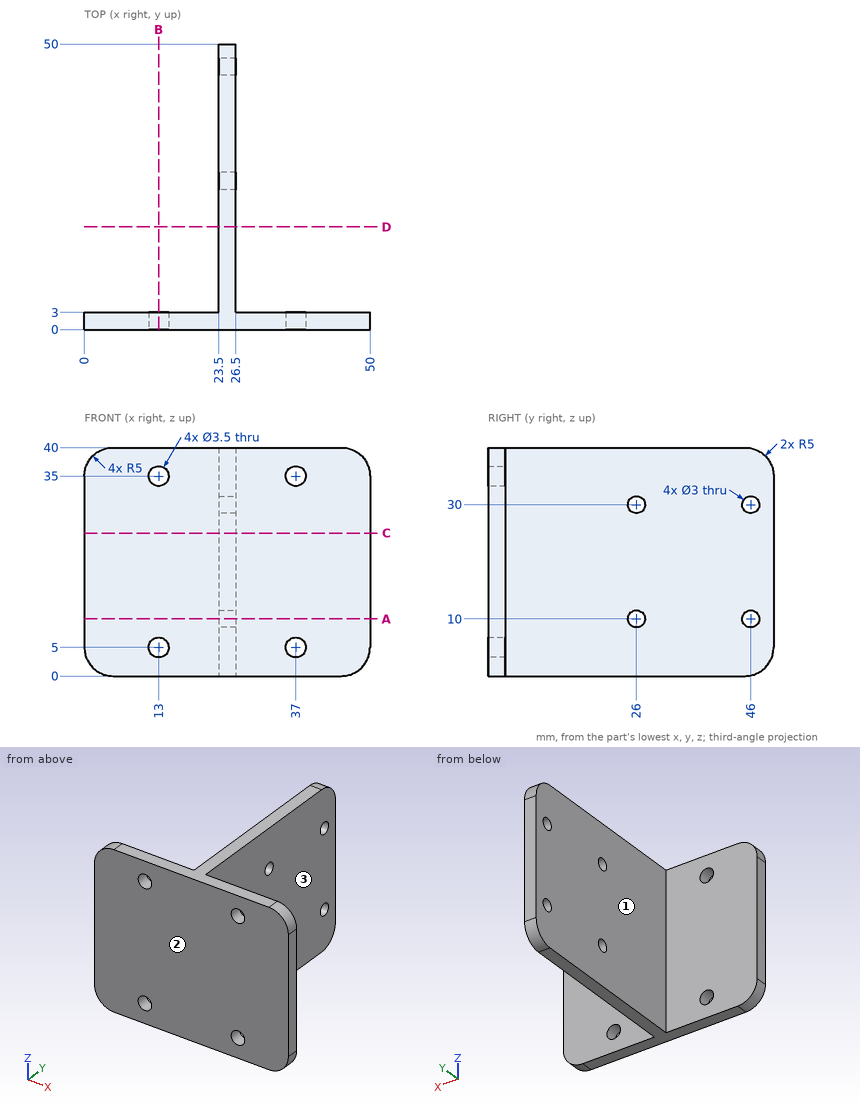
Job drawing, mm, ordinate dimensions from the low corner. One solid piece. A direction names the side the tool comes from. Give positions to 0.01 mm unless a question says otherwise; leave off trailing zeros. Loops run counter-clockwise (first coordinate to the right, second up) from the corner with the lowest first, then second, coordinate; pieces in that order, holes last.
Item 1: Slice it at B-B, the plane x = 13. List the corners of the cut face in (y, z), and give its area (3 significant figures).
Answers follow:
outline: (0, 0) - (3, 0) - (3, 3.25) - (0, 3.25) - close; (0, 6.75) - (3, 6.75) - (3, 33.25) - (0, 33.25) - close; (0, 36.75) - (3, 36.75) - (3, 40) - (0, 40) - close
area: 99.0 mm2
Item 2: Drill centre lines: line 1 (Y direction, x = 25, z = 30); line 2 (Y direction, x = 5, z = 13); line 3 (X direction, y = 40.5, z = 8.5). Where is each one in solid material? Low to high.
Answers follow:
line 1: y = 0 to 24.5, 27.5 to 44.5, 47.5 to 50
line 2: y = 0 to 3
line 3: x = 23.5 to 26.5
Item 3: Which spindle directions (+Z, -Z, +X, -X, +Y, -Y) get a long thin tool onto all of the face, cutting with end or side? Do the marked faces 1, 2 and 3. Say none if no direction does.
Answers follow:
face 1: +Z, -Z, -X, +Y
face 2: +Z, -Z, +X, -X, -Y
face 3: +Z, -Z, +X, +Y
Item 4: Flat gauge pins, fed straight in: pin 1 (12 mm diameter, centred on y = 24.5, z = 24.5, fed in from +X); pin 2 (1.5 mm diameter, centred on y = 8.5, z = 10.5, fed in from -X); pin 3 (2 mm diameter, centred on x = 17.5, z = 36, fed in from +Y); pin 4 (1.8 mm diameter, centred on y = 26, z = 30, fed in from +X). Where does each tip first touch, or does it go through?
Answers follow:
pin 1: stops at x = 26.5
pin 2: stops at x = 23.5
pin 3: stops at y = 3
pin 4: passes through
Item 5: Slice it at C-C, the plane z = 25. List the corners of the cut face in (x, y).
Answers follow:
outline: (0, 0) - (50, 0) - (50, 3) - (26.5, 3) - (26.5, 50) - (23.5, 50) - (23.5, 3) - (0, 3) - close
Item 6: Slice it at D-D, the plane y = 18. List the corners of the cut face in (x, z), and give its area (3 significant figures).
Answers follow:
outline: (23.5, 0) - (26.5, 0) - (26.5, 40) - (23.5, 40) - close
area: 120 mm2
Item 7: Slice it at A-A, the plane z = 10. List the corners of the cut face in (x, y), and give its area (3 significant figures).
Answers follow:
outline: (0, 0) - (50, 0) - (50, 3) - (26.5, 3) - (26.5, 24.5) - (23.5, 24.5) - (23.5, 3) - (0, 3) - close; (23.5, 27.5) - (26.5, 27.5) - (26.5, 44.5) - (23.5, 44.5) - close; (23.5, 47.5) - (26.5, 47.5) - (26.5, 50) - (23.5, 50) - close
area: 273 mm2
